Here's how the part is built. I have some questions about the finished solid (model axes, mm). Round coordinates to 2 decimals unless told otherwise and drop trailing zeros. Write each loop counter-clockwise with the first axis right and the second up, starting at its lowest first coordinate (ties: lowest second). Pieces come first, ordered by that corner, then holes. Notation, with made-up numbers: (23.25, 37) - (47.25, 37) arc R14 cw to (47.25, 48) - close; hole circle Ø9 at (44, 39.5). An arc over 180 degrees is marked (long way). Write item = value, one per line. Start each with the question number.
Item 1: If we section it at A-A (x = 1180): Please give me the cut outline in (y, z), and give its area (3 significant figures).
Item 2: If we section it at B-B (z = -67): Please give me the cut outline in (x, y), and give its area (3 significant figures).
Item 3: If I drill on line 1 along Z through (x, y) = (1237.5, 11); line 2 along Y through (x, z) = (1556, -52); line 3 along Y through (x, z) = (1339.5, -84), over which ranges is the centre line in solid material (lowest first)? Write a range as [from, to].
Item 4: If we section it at C-C (y = 54): Please give me the cut outline in (x, z).
Item 5: Thinking about a two-plate mould opening in Y: for faces 1 (the face through (1137, 40, -85)), 2 (the face through (1137, -3, -43)), 3 (the face through (1139, 42, -88)), 4 (the face through (1136, 0, -40)), which applies, pulls with the +Y half, pulls with the -Y half, needs draft (parallel to the pull), parting line crosses it, or undercut?
Item 6: For P1, Ø3, axis at x = 1920.5, z = -34, coming from the +Y side; P2, Ø12, axis at y = 7.5, z = -48.5, coming from the +X side, each with a flat end and sliding along its axis, tell me the tip position at first contact or that it passes through.
```python
from build123d import *

# Parameters (mm, degrees)
BOSS_EXTRUDE1_DEPTH     = 2310
FILLET1_R               = 3
CUT_EXTRUDE1_DEPTH      = 85
CUT_EXTRUDE1_DEPTH_BACK = 2315.387175906
SKETCH6_W               = 2310
SKETCH6_H               = 30
CUT_EXTRUDE2_DEPTH      = 41


with BuildPart() as part:
    # Sketch1 → Boss-Extrude1 (new body)
    with BuildSketch(Plane(origin=(0, 0, 0), x_dir=(0, 0, -1), z_dir=(1, 0, 0))):
        Polygon((0, 0), (85, 0), (85, 82), (47, 82), (47, 112), (50, 112), (50, 85), (88, 85), (88, -3), (0, -3), align=None)
    extrude(amount=BOSS_EXTRUDE1_DEPTH)

    # Fillet1
    fillet1_edges = [part.edges().sort_by_distance(p)[0] for p in [
        (1155, 0, -85),
        (1155, 82, -85),
        (1155, 82, -47),
        (1155, 85, -50),
        (1155, 85, -88),
        (1155, -3, -88),
    ]]
    fillet(fillet1_edges, radius=FILLET1_R)

    # Sketch3 → Cut-Extrude1 (cut, two sides: drawn at the far end of the back side and taken through both)
    with BuildSketch(Plane(origin=(0, 0, 0), x_dir=(1, 0, 0), z_dir=(0, 1, 0)).offset(-CUT_EXTRUDE1_DEPTH_BACK)):
        Polygon((2310, 88), (2222, 0), (2310, 0), align=None)
    extrude(amount=CUT_EXTRUDE1_DEPTH + CUT_EXTRUDE1_DEPTH_BACK, mode=Mode.SUBTRACT)

    # Sketch6 → Cut-Extrude2 (cut)
    with BuildSketch(Plane.XY.offset(-47)):
        with Locations((1155, 97)):
            Rectangle(SKETCH6_W, SKETCH6_H)
    extrude(amount=-CUT_EXTRUDE2_DEPTH, mode=Mode.SUBTRACT)


solid = part.part
```
Reply:
q1.outline = (-3, -85) arc R3 ccw to (0, -88) - (82, -88) - (82, -82) arc R3 cw to (79, -85) - (3, -85) arc R3 cw to (0, -82) - (0, 0) - (-3, 0) - close
q1.area = 512 mm2
q2.outline = (0, -3) - (2289, -3) - (2289, 0) - (0, 0) - close
q2.area = 6,870 mm2
q3.line_1 = [-88, -85]
q3.line_2 = [-3, 0]
q3.line_3 = [-3, 0.76], [81.24, 82]
q4.outline = (0, -88) - (2310, -88) - (2307, -85) - (0, -85) - close
q5.face_1 = undercut
q5.face_2 = pulls with the -Y half
q5.face_3 = needs draft
q5.face_4 = pulls with the +Y half
q6.P1 = 0
q6.P2 = through
